from build123d import *

# Parameters (mm, degrees)
SKETCH1_W                        = 125
SKETCH1_H                        = 120
TEST_BASE_POSTION_DEPTH          = 11.215
SKETCH10_R                       = 15.25
CONNECT_FINGER_HOLES_DEPTH       = 98.597363925
SKETCH11_R                       = 18.5
XL320_FINGER_KNUCKLE_MOUNT_DEPTH = 6.6025
SKETCH24_R                       = 2.25
AX12_MOUNT_HOLES_M4_DEPTH        = 98.597363925
SKETCH21_R                       = 17.65
SKETCH21_R_2                     = 10.15
GEARS_HOLES_DEPTH                = 6.6025
SKETCH22_R                       = 1.15
GEARS_ROD_HOLES_DEPTH            = 3
CUT_EXTRUDE1_DEPTH               = 98.597363925
FILLET1_R                        = 10
SKETCH17_R                       = 3.25
CONNECT_HOLES_M6_DEPTH           = 98.597363925
NUTS_M6_DEPTH                    = 6
NUTS_M4_DEPTH                    = 5
SKETCH30_R                       = 2
CONNECT_TO_HOUSE_DEPTH           = 98.597363925
SKETCH31_R                       = 2.25
M4_EXTENSION_HOLE_DEPTH          = 5
SKETCH28_R                       = 1
M2_SHAFT_HOLE_DEPTH              = 3


with BuildPart() as part:
    # Sketch1 → Test_Base_Postion (new body)
    with BuildSketch(Plane(origin=(0, 0, 0), x_dir=(1, 0, 0), z_dir=(0, 1, 0))):
        with BuildLine():
            ThreePointArc((-62.5, 60), (-76.154246239, 0), (-62.5, -60))
            Line((-62.5, -60), (-62.5, 60))
        make_face()
        Rectangle(SKETCH1_W, SKETCH1_H)
    extrude(amount=TEST_BASE_POSTION_DEPTH)

    # Sketch10 → Connect_Finger_Holes (cut, through all)
    with BuildSketch(Plane(origin=(0, 11.215, 0), x_dir=(1, 0, 0), z_dir=(0, 1, 0))):
        with Locations(Location((-36.5, 30, 0), (0, 0, 270))):
            Circle(SKETCH10_R)
        with Locations(Location((-36.5, -30, 0), (0, 0, 270))):
            Circle(SKETCH10_R)
        with Locations(Location((42, 0, 0), (0, 0, 270))):
            Circle(SKETCH10_R)
    extrude(amount=-CONNECT_FINGER_HOLES_DEPTH, mode=Mode.SUBTRACT)

    # Sketch11 → XL320_Finger_Knuckle_Mount (cut)
    with BuildSketch(Plane(origin=(0, 11.215, 0), x_dir=(1, 0, 0), z_dir=(0, 1, 0))):
        with Locations(Location((42, 0, 0), (0, 0, 270))):
            Circle(SKETCH11_R)
    extrude(amount=-XL320_FINGER_KNUCKLE_MOUNT_DEPTH, mode=Mode.SUBTRACT)

    # Sketch24 → AX12_Mount_Holes_(M4) (cut, through all)
    with BuildSketch(Plane(origin=(0, 11.215, 0), x_dir=(1, 0, 0), z_dir=(0, 1, 0))):
        with Locations(Location((9.75, 52.25, 0), (0, 0, 270))):
            Circle(SKETCH24_R)
        with Locations(Location((0.75, 20.25, 0), (0, 0, 270))):
            Circle(SKETCH24_R)
        with Locations(Location((0.75, -20.25, 0), (0, 0, 270))):
            Circle(SKETCH24_R)
        with Locations(Location((9.75, -52.25, 0), (0, 0, 270))):
            Circle(SKETCH24_R)
        with Locations(Location((10.75, 40, 0), (0, 0, 270))):
            Circle(SKETCH24_R)
        with Locations(Location((31.25, 49, 0), (0, 0, 270))):
            Circle(SKETCH24_R)
    extrude(amount=-AX12_MOUNT_HOLES_M4_DEPTH, mode=Mode.SUBTRACT)

    # Sketch21 → Gears_Holes (cut)
    with BuildSketch(Plane(origin=(0, 11.215, 0), x_dir=(1, 0, 0), z_dir=(0, 1, 0))):
        with Locations((-36.5, 30)):
            Circle(SKETCH21_R)
        with Locations((-23.330432809, 8.75)):
            Circle(SKETCH21_R_2)
        with Locations((-23.330432809, -8.75)):
            Circle(SKETCH21_R_2)
        with Locations((-36.5, -30)):
            Circle(SKETCH21_R)
    extrude(amount=-GEARS_HOLES_DEPTH, mode=Mode.SUBTRACT)

    # Sketch22 → Gears_Rod_Holes (cut)
    with BuildSketch(Plane(origin=(0, 4.6125, 0), x_dir=(1, 0, 0), z_dir=(0, 1, 0))):
        with Locations(Location((-23.330432809, -8.75, 0), (0, 0, 270))):
            Circle(SKETCH22_R)
    extrude(amount=-GEARS_ROD_HOLES_DEPTH, mode=Mode.SUBTRACT)

    # Sketch29 → Cut-Extrude1 (cut, through all)
    with BuildSketch(Plane(origin=(0, 11.215, 0), x_dir=(1, 0, 0), z_dir=(0, 1, 0))):
        Polygon((27.5, 60), (62.5, 40), (62.5, 60), align=None)
        Polygon((62.5, -60), (27.5, -60), (62.5, -40), align=None)
    extrude(amount=-CUT_EXTRUDE1_DEPTH, mode=Mode.SUBTRACT)

    # Fillet1
    fillet1_edges = [part.edges().sort_by_distance(p)[0] for p in [
        (62.5, 5.6075, 40),
        (27.5, 5.6075, 60),
        (-62.5, 5.6075, -60),
        (-62.5, 5.6075, 60),
        (27.5, 5.6075, -60),
        (62.5, 5.6075, -40),
    ]]
    fillet(fillet1_edges, radius=FILLET1_R)

    # Sketch17 → Connect_Holes_(M6) (cut, through all)
    with BuildSketch(Plane(origin=(0, 11.215, 0), x_dir=(1, 0, 0), z_dir=(0, 1, 0))):
        with Locations(Location((-58.040773893, 51.152938298, 0), (0, 0, 270))):
            Circle(SKETCH17_R)
        with Locations(Location((-58.040773893, -51.152938298, 0), (0, 0, 270))):
            Circle(SKETCH17_R)
        with Locations(Location((28.844355629, -51.794444289, 0), (0, 0, 270))):
            Circle(SKETCH17_R)
    extrude(amount=-CONNECT_HOLES_M6_DEPTH, mode=Mode.SUBTRACT)

    # Sketch19 → Nuts_(M6) (cut)
    with BuildSketch(Plane.XZ):
        Polygon((-58.040773893, 56.92644099), (-63.040773893, 54.039689644), (-63.040773893, 48.266186952), (-58.040773893, 45.379435606), (-53.040773893, 48.266186952), (-53.040773893, 54.039689644), align=None)
        Polygon((28.844355629, 57.56794698), (23.844355629, 54.681195634), (23.844355629, 48.907692943), (28.844355629, 46.020941597), (33.844355629, 48.907692943), (33.844355629, 54.681195634), align=None)
        Polygon((-58.040773893, -45.379435606), (-63.040773893, -48.266186952), (-63.040773893, -54.039689644), (-58.040773893, -56.92644099), (-53.040773893, -54.039689644), (-53.040773893, -48.266186952), align=None)
    extrude(amount=-NUTS_M6_DEPTH, mode=Mode.SUBTRACT)

    # Sketch27 → Nuts_(M4) (cut)
    with BuildSketch(Plane.XZ):
        Polygon((9.75, 56.291451884), (6.25, 54.270725942), (6.25, 50.229274058), (9.75, 48.208548116), (13.25, 50.229274058), (13.25, 54.270725942), align=None)
        Polygon((-2.75, 22.270725942), (-2.75, 18.229274058), (0.75, 16.208548116), (4.25, 18.229274058), (4.25, 22.270725942), (0.75, 24.291451884), align=None)
        Polygon((-2.75, -22.270725942), (0.75, -24.291451884), (4.25, -22.270725942), (4.25, -18.229274058), (0.75, -16.208548116), (-2.75, -18.229274058), align=None)
        Polygon((6.25, -50.229274058), (6.25, -54.270725942), (9.75, -56.291451884), (13.25, -54.270725942), (13.25, -50.229274058), (9.75, -48.208548116), align=None)
        Polygon((14.25, -37.979274058), (10.75, -35.958548116), (7.25, -37.979274058), (7.25, -42.020725942), (10.75, -44.041451884), (14.25, -42.020725942), align=None)
        Polygon((27.75, -46.979274058), (27.75, -51.020725942), (31.25, -53.041451884), (34.75, -51.020725942), (34.75, -46.979274058), (31.25, -44.958548116), align=None)
    extrude(amount=-NUTS_M4_DEPTH, mode=Mode.SUBTRACT)

    # Sketch30 → Connect_To_House (cut, through all)
    with BuildSketch(Plane(origin=(0, 11.215, 0), x_dir=(1, 0, 0), z_dir=(0, 1, 0))):
        with Locations(Location((2.5, 0, 0), (0, 0, 270))):
            Circle(SKETCH30_R)
    extrude(amount=-CONNECT_TO_HOUSE_DEPTH, mode=Mode.SUBTRACT)

    # Sketch31 → M4_Extension_Hole (cut)
    with BuildSketch(Plane(origin=(0, 11.215, 0), x_dir=(1, 0, 0), z_dir=(0, 1, 0))):
        with Locations(Location((-62.75, 19.41386581, 0), (0, 0, 270))):
            Circle(SKETCH31_R)
        with Locations(Location((-62.75, 7.41386581, 0), (0, 0, 270))):
            Circle(SKETCH31_R)
        with Locations(Location((36, -24, 0), (0, 0, 270))):
            Circle(SKETCH31_R)
        with Locations(Location((48, -24, 0), (0, 0, 270))):
            Circle(SKETCH31_R)
    extrude(amount=-M4_EXTENSION_HOLE_DEPTH, mode=Mode.SUBTRACT)

    # Sketch28 → M2_Shaft_Hole (cut)
    with BuildSketch(Plane(origin=(0, 4.6125, 0), x_dir=(1, 0, 0), z_dir=(0, 1, 0))):
        with Locations(Location((-23.330432809, 8.75, 0), (0, 0, 270))):
            Circle(SKETCH28_R)
    extrude(amount=-M2_SHAFT_HOLE_DEPTH, mode=Mode.SUBTRACT)


solid = part.part
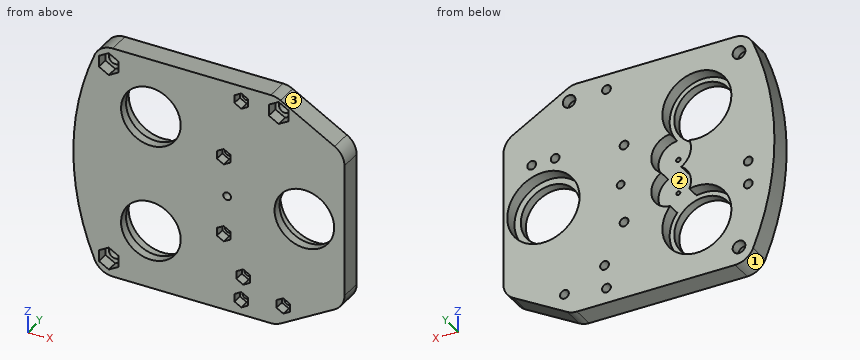
Could you check a few things on this model? Use its own coordinates, in mm. Face numbers are marked on the shaded views. Round coordinates to 2 decimals unless told otherwise and drop trailing zeros. Write each loop counter-clockwise with the first axis right and the second up, starting at its lowest first coordinate (ties: lowest second). Pieces come first, ordered by that corner, then holes. Notation, with made-up numbers: (73, -6.75) - (104, -6.75) arc R27 cw to (104, 20.25) - close; hole circle Ø2 at (-40, 72). An arc over 180 degrees is marked (long way). Put each result on its own line as item: value. Start each with the question number.
(1) I need wall thicknesses on probe 1 along X at (y, z) = (3.6, 0); probe 2 along Z at (x, y) = (-36.5, 10.5); probe 3 along Z at (x, y) = (-32.5, 4). Which ranges of each line are inside material? Lowest first, please.
(2) I want a section at B-B, the plane z = -29.5. Please give me the cut outline in (x, y) (1 decimal).
(3) I want a section at D-D, the plane z = 40.5. Please give me the cut outline in (x, y) (1 decimal).
(4) Will these pins go through, and if not, where does the flat tip stop? pin 1 (2 mm diameter, centred on x = -63.5, z = -6.5, fed in from +Y) (3 decimals); pin 2 (4.5 mm diameter, centred on y = 2, z = -39, fed in from +X); pin 3 (3.5 mm diameter, centred on x = 10.5, z = 52, fed in from -Y).
(5) I want a section at A-A, the plane x = -36.5. Give the number of separate pieces and of enclosed holes in the cut face, plus the area to 3 significant figures.
(6) Thinking about a two-plate mould opening in X: for the marked faces 1, 2 and 3, which applies, released by +X, released by -X, zero draft, split by the parting line, or undercut?
Here are the results:
1. probe 1: x = -76.15 to 0.5, 4.5 to 26.75, 57.25 to 62.5
1. probe 2: z = -60 to -47.65, -12.35 to 12.35, 47.65 to 60
1. probe 3: z = -60 to -44.72, -15.28 to 15.28, 44.72 to 60
2. outline: (-73, 0) - (-51.7, 0) - (-51.7, 4.6) - (-54.1, 4.6) - (-54.1, 11.2) - (-73, 11.2) - close; (-21.3, 0) - (62.5, 0) - (62.5, 11.2) - (-18.9, 11.2) - (-18.9, 4.6) - (-21.3, 4.6) - close
3. outline: (-70.1, 0) - (-47.6, 0) - (-47.6, 4.6) - (-50.7, 4.6) - (-50.7, 11.2) - (-70.1, 11.2) - close; (-25.4, 0) - (60.3, 0) - (60.3, 11.2) - (-22.3, 11.2) - (-22.3, 4.6) - (-25.4, 4.6) - close
4. pin 1: stops at y = 6.215
4. pin 2: stops at x = 62.17
4. pin 3: stops at y = 5
5. separate pieces: 3
5. enclosed holes: 0
5. area: 598 mm^2
6. face 1: released by -X
6. face 2: undercut
6. face 3: released by +X
